```python
from build123d import *

# Parameters (mm, degrees)
F0_W      = 42
F0_H      = 42.35
F1_DEPTH  = 4.2
F2_R      = 11
F2_R_2    = 1.6
F3_DEPTH  = 4.201
F4_W      = 9.35
F4_H      = 42.35
F5_DEPTH  = 12.6
F6_R      = 1.6
F7_DEPTH  = 16.801
F8_R      = 3
F9_DEPTH  = 2.7
F10_R     = 3
F11_DEPTH = 2.2
F12_R     = 4
F13_R     = 2.5
F14_R     = 1.5
F14_R_2   = 3
F15_DEPTH = 42.001
F16_R     = 3
F17_DEPTH = 2.5


with BuildPart() as f1:
    # F0 (on Right) → F1 (new body)
    with BuildSketch(Plane.YZ):
        Rectangle(F0_W, F0_H)
    extrude(amount=F1_DEPTH)

    # F2 (on face) → F3 (cut, through all)
    with BuildSketch(Plane.YZ.offset(4.2)):
        Circle(F2_R)
        with Locations((15.8, 15.5)):
            Circle(F2_R_2)
        with Locations((15.8, -15.5)):
            Circle(F2_R_2)
    extrude(amount=-F3_DEPTH, mode=Mode.SUBTRACT)

    # F4 (on face) → F5 (join)
    with BuildSketch(Plane.YZ.offset(4.2)):
        with Locations((-16.325, 0)):
            Rectangle(F4_W, F4_H)
    extrude(amount=F5_DEPTH)

    # F6 (on face) → F7 (cut, through all)
    with BuildSketch(Plane.YZ.offset(16.8)):
        with Locations((-15.2, 15.5)):
            Circle(F6_R)
        with Locations((-15.2, -15.5)):
            Circle(F6_R)
    extrude(amount=-F7_DEPTH, mode=Mode.SUBTRACT)

    # F8 (on face) → F9 (cut)
    with BuildSketch(Plane.YZ.offset(16.8)):
        with Locations((-15.2, -15.5)):
            Circle(F8_R)
        with Locations((-15.2, 15.5)):
            Circle(F8_R)
    extrude(amount=-F9_DEPTH, mode=Mode.SUBTRACT)

    # F10 (on face) → F11 (cut)
    with BuildSketch(Plane.YZ.offset(4.2)):
        with Locations((15.8, 15.5)):
            Circle(F10_R)
    extrude(amount=-F11_DEPTH, mode=Mode.SUBTRACT)

    # F12
    f12_edges = [f1.edges().sort_by_distance(p)[0] for p in [
        (2.1, 21, 21.175),
        (2.1, 21, -21.175),
    ]]
    fillet(f12_edges, radius=F12_R)

    # F13
    f13_edges = [f1.edges().sort_by_distance(p)[0] for p in [
        (10.5, -11.65, 21.175),
        (10.5, -11.65, -21.175),
        (8.4, -21, 21.175),
        (8.4, -21, -21.175),
    ]]
    fillet(f13_edges, radius=F13_R)

    # F14 (on face) → F15 (cut, through all)
    with BuildSketch(Plane.XZ.offset(21)):
        with Locations((10.3, 10.425)):
            Circle(F14_R)
        with Locations((10.3, -6.075)):
            Circle(F14_R_2)
    extrude(amount=-F15_DEPTH, mode=Mode.SUBTRACT)

    # F16 (on face) → F17 (cut)
    with BuildSketch(Plane.XZ.offset(21)):
        with Locations((10.3, 10.425)):
            Circle(F16_R)
    extrude(amount=-F17_DEPTH, mode=Mode.SUBTRACT)


solid = f1.part
```
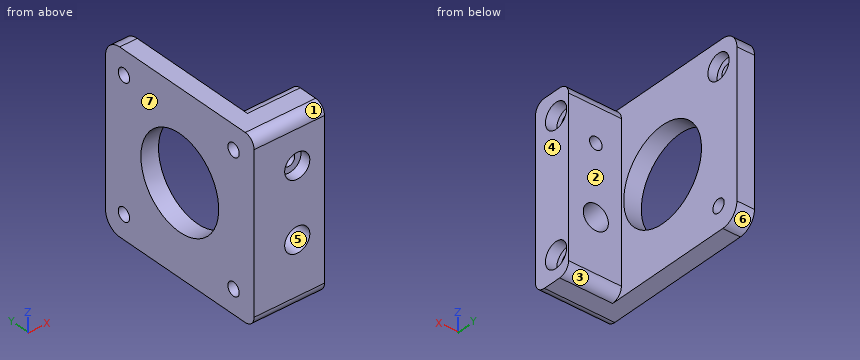
CAD build for the part. Positions are in the model's coordinates, mm. Face numbers are marked on the shaded views. A direction names the side the tool comes from. Give positions to 0.01 mm unless a question says otherwise; leave off trailing zeros. Order: outer loops, then holes, each group sorted by start corner. A loop starts at its lowest first (then second) coordinate and runs counter-clockwise, first axis right, second up.
(1) Mould opens along X. For the marked faces 4, 5, 6 and 7 say: released by +X, released by -X, zero draft, split by the parting line, or undercut.
(2) Drill centre lines: L1, parallel to Z at x = 15.05, y = -15.2 (3 decimals); L2, parallel to X at y = -14.5, z = -6; L3, parallel to Z at x = 10.3, y = -19.85 (3 decimals). Where is each one in solid material? Low to high.
(3) Saw through at A-A, the plane y = 15.8. Give the cut face in (x, z) (3 decimals), then the cut area to 3 significant figures.
(4) Saw through at D-D, the plane z = -15.5. Give the cut face in (x, y), then the cut area to 3 significant figures.
(5) Saw through at B-B, the plane x = 10.3. Give the cut face in (y, z) (3 decimals), then the cut area to 3 significant figures.
(6) Tool access for the marked faces 1, 2 and 3: list every direction of +Z, -Z, +X, -X, +Y, -Y with a clear straight run to the whole face (end or side of a thin tool).
(7) Flat gauge pins, fed straight in: pin 1 (1.5 mm diameter, centred on x = 6.5, z = 9, fed in from +Y); pin 2 (2.5 mm diameter, centred on y = 15.8, z = -15.5, fed in from +X); pin 3 (4 mm diameter, centred on y = -15.2, z = 15.5, fed in from +X); pin 4 (3.5 mm diameter, centred on y = 15.8, z = 15.5, fed in from +X). Where does each tip first touch, or does it go through?
(8) Saw through at C-C, the plane x = 5.25. Give the cut face in (y, z) (3 decimals).
Results found:
1. face 4: released by +X
1. face 5: undercut
1. face 6: zero draft
1. face 7: released by -X
2. L1: z = -21.175 to -18.5, -12.5 to 12.5, 18.5 to 21.175
2. L2: x = 0 to 7.3, 13.3 to 16.8
2. L3: z = -20.779 to -9.075, -3.075 to 7.425, 13.425 to 20.779
3. outline: (0, -21.175) - (4.2, -21.175) - (4.2, -17.1) - (0, -17.1) - close; (0, -13.9) - (4.2, -13.9) - (4.2, 12.5) - (2, 12.5) - (2, 13.9) - (0, 13.9) - close; (0, 17.1) - (2, 17.1) - (2, 18.5) - (4.2, 18.5) - (4.2, 21.175) - (0, 21.175) - close
3. area: 145 mm2
4. outline: (0, -21) - (16.8, -21) - (16.8, -18.2) - (14.1, -18.2) - (14.1, -16.8) - (0, -16.8) - close; (0, -13.6) - (14.1, -13.6) - (14.1, -12.2) - (16.8, -12.2) - (16.8, -11.65) - (4.2, -11.65) - (4.2, 14.2) - (0, 14.2) - close; (0, 17.4) - (4.2, 17.4) - (4.2, 21) - (0, 21) - close
4. area: 219 mm2
5. outline: (-21, -18.675) arc R2.5 ccw to (-18.5, -21.175) - (-14.15, -21.175) arc R2.5 ccw to (-11.65, -18.675) - (-11.65, -9.075) - (-21, -9.075) - close; (-21, -3.075) - (-11.65, -3.075) - (-11.65, 8.925) - (-18.5, 8.925) - (-18.5, 7.425) - (-21, 7.425) - close; (-21, 13.425) - (-18.5, 13.425) - (-18.5, 11.925) - (-11.65, 11.925) - (-11.65, 18.675) arc R2.5 ccw to (-14.15, 21.175) - (-18.5, 21.175) arc R2.5 ccw to (-21, 18.675) - close; hole circle Ø3.2 at (-15.2, -15.5); hole circle Ø3.2 at (-15.2, 15.5)
5. area: 283 mm2
6. face 1: +Z, +X, -X, -Y
6. face 2: +Z, -Z, +X, +Y
6. face 3: -Z, +X, +Y
7. pin 1: stops at y = -11.65
7. pin 2: passes through
7. pin 3: stops at x = 14.1
7. pin 4: stops at x = 2
8. outline: (-21, -18.675) arc R2.5 ccw to (-18.5, -21.175) - (-14.15, -21.175) arc R2.5 ccw to (-11.65, -18.675) - (-11.65, 18.675) arc R2.5 ccw to (-14.15, 21.175) - (-18.5, 21.175) arc R2.5 ccw to (-21, 18.675) - close; hole circle Ø3.2 at (-15.2, -15.5); hole circle Ø3.2 at (-15.2, 15.5)
